```python
from build123d import *

# Parameters (mm, degrees)
SKETCH1_R           = 2.1
SKETCH1_R_2         = 6
SKETCH1_R_3         = 11
SKETCH1_R_4         = 1.6
SKETCH1_R_5         = 2
BOSS_EXTRUDE1_DEPTH = 8


with BuildPart() as part:
    # Sketch1 → Boss-Extrude1 (new body)
    with BuildSketch(Plane.XY):
        with BuildLine():
            Line((-58.658661762, -94.325772402), (11.341338238, -94.325772402))
            ThreePointArc((11.341338238, -94.325772402), (14.876872144, -92.861306308), (16.341338238, -89.325772402))
            Line((16.341338238, -89.325772402), (16.341338238, -55.206132823))
            ThreePointArc((16.341338238, -55.206132823), (18.853727353, -43.188177597), (25.970088092, -33.18314103))
            Line((25.970088092, -33.18314103), (78.712588384, 15.603630397))
            ThreePointArc((78.712588384, 15.603630397), (85.828949123, 25.608666964), (88.341338238, 37.62662219))
            Line((88.341338238, 37.62662219), (88.341338238, 93.338561628))
            ThreePointArc((88.341338238, 93.338561628), (82.483473862, 107.480697252), (68.341338238, 113.338561628))
            Line((68.341338238, 113.338561628), (46.341338238, 113.338561628))
            ThreePointArc((46.341338238, 113.338561628), (32.199202614, 107.480697252), (26.341338238, 93.338561628))
            Line((26.341338238, 93.338561628), (26.341338238, 65.996620638))
            ThreePointArc((26.341338238, 65.996620638), (23.98166612, 54.334190592), (17.273853267, 44.506394613))
            Line((17.273853267, 44.506394613), (-54.591176791, -25.493605387))
            ThreePointArc((-54.591176791, -25.493605387), (-61.298989644, -35.321401365), (-63.658661762, -46.983831411))
            Line((-63.658661762, -46.983831411), (-63.658661762, -89.325772402))
            ThreePointArc((-63.658661762, -89.325772402), (-62.194195668, -92.861306308), (-58.658661762, -94.325772402))
        make_face()
        with Locations((-56.658661762, -57.075772402)):
            Circle(SKETCH1_R, mode=Mode.SUBTRACT)
        with Locations((-30.658661762, -57.075772402)):
            Circle(SKETCH1_R, mode=Mode.SUBTRACT)
        with Locations((-30.658661762, -87.575772402)):
            Circle(SKETCH1_R, mode=Mode.SUBTRACT)
        with Locations((-56.658661762, -87.575772402)):
            Circle(SKETCH1_R, mode=Mode.SUBTRACT)
        with Locations((9.341338238, -87.575772402)):
            Circle(SKETCH1_R, mode=Mode.SUBTRACT)
        with Locations((-16.658661762, -87.575772402)):
            Circle(SKETCH1_R, mode=Mode.SUBTRACT)
        with Locations((-16.658661762, -57.075772402)):
            Circle(SKETCH1_R, mode=Mode.SUBTRACT)
        with Locations((9.341338238, -57.075772402)):
            Circle(SKETCH1_R, mode=Mode.SUBTRACT)
        with Locations((57.341338238, 99.338561628)):
            Circle(SKETCH1_R_2, mode=Mode.SUBTRACT)
        with Locations((57.341338238, 27.398561628)):
            Circle(SKETCH1_R_2, mode=Mode.SUBTRACT)
        with Locations((57.341338238, 63.368561628)):
            Circle(SKETCH1_R_3, mode=Mode.SUBTRACT)
        with Locations((41.841338238, 78.868561628)):
            Circle(SKETCH1_R_4, mode=Mode.SUBTRACT)
        with Locations((72.841338238, 78.868561628)):
            Circle(SKETCH1_R_4, mode=Mode.SUBTRACT)
        with Locations((72.841338238, 47.868561628)):
            Circle(SKETCH1_R_4, mode=Mode.SUBTRACT)
        with Locations((41.841338238, 47.868561628)):
            Circle(SKETCH1_R_4, mode=Mode.SUBTRACT)
        with Locations((84.341338238, 37.62662219)):
            Circle(SKETCH1_R_5, mode=Mode.SUBTRACT)
        with Locations((84.351781192, 88.518513838)):
            Circle(SKETCH1_R_5, mode=Mode.SUBTRACT)
        with Locations((47.341338238, 99.338561628)):
            Circle(SKETCH1_R_4, mode=Mode.SUBTRACT)
        with Locations((47.341338238, 27.398561628)):
            Circle(SKETCH1_R_4, mode=Mode.SUBTRACT)
        with Locations((67.341338238, 99.338561628)):
            Circle(SKETCH1_R_4, mode=Mode.SUBTRACT)
        with Locations((67.341338238, 27.398561628)):
            Circle(SKETCH1_R_4, mode=Mode.SUBTRACT)
        with Locations((84.346559715, 63.072568014)):
            Circle(SKETCH1_R_5, mode=Mode.SUBTRACT)
    extrude(amount=BOSS_EXTRUDE1_DEPTH)


solid = part.part
```
Source: CAD feature listing. Evaluate the final solid. Frame: model axes, mm. A direction names the side the tool comes from. Coordinates: 2 decimals unless noted, no trailing zeros. Loops run counter-clockwise (first coordinate to the right, second up) from the corner with the lowest first, then second, coordinate; pieces in that order, holes last. Notation, with made-up numbers: M -17,-11.5 L 42,-11.5 A7 cw 42,-4.5 Z; hole C 28.5,49.5 d3. An arc over 180 degrees is marked long. Put each result on its own line as item: value. Start each with the question number.
1) Cut plane B-B on x = 53.5. Return the cut outline in (y, z), then the cut area to 3 significant figures.
2) Ray query, L1, parallel to Y at x = 66, z = 3; L2, parallel to Y at x = 56, z = 5; L3, parallel to Y at x = -31.5, z = 0.5. Return the intervals inside material, ascending. Write a range as from..to.
3) Contact query for flat-ended pins moving along their axis: pin 1 Ø3 at (x, y) = (47.34, 99.34) entering from +Z; pin 2 Ø4 at (y, z) = (85, 2) entering from -X. Output: stop coordinate, or through.
4) Pull-direction query (X, two-part tool) for faces 1 (the face through (52.919, 103.394, 3.944)), 2 (the face through (11, 11, 0)), 3 (the face through (-63.659, -68, 4)); classes: pulls with the +X half, pulls with the -X half, needs draft (parallel to the pull), parting line crosses it, or undercut.
5) Cut plane D-D on z = 6.5. Give the number of separate pieces and of enclosed holes in the cut face, then the cut area to 3 significant figures.
6) Reachability of faces 4 (the face through (26.341, 80, 4)), 5 (the face through (83.91, 61.12, 3.94)) from +Z, -Z, +X, -X, +Y, -Y: full face, straight path, thin tool, end or side. Return the list, or none.
7) Cut plane A-A on y = 70.5. Return the cut outline in (x, z).
8) Cut plane C-C on y = -71. Return the cut outline in (x, z).
The answers:
1. outline: M -7.72,0 L 22.79,0 L 22.79,8 L -7.72,8 Z; M 32.01,0 L 53.06,0 L 53.06,8 L 32.01,8 Z; M 73.68,0 L 94.73,0 L 94.73,8 L 73.68,8 Z; M 103.95,0 L 113.34,0 L 113.34,8 L 103.95,8 Z
1. area: 656 mm²
2. L1: y = 3.84..26.53, 28.27..56.58, 70.15..98.47, 100.21..113.34
2. L2: y = -5.41..21.55, 33.25..52.45, 74.29..93.49, 105.19..113.34
2. L3: y = -94.33..-89.5, -85.65..-59, -55.15..-3
3. pin 1: passes through
3. pin 2: stops at x = 26.34
4. face 1: undercut
4. face 2: needs draft
4. face 3: pulls with the -X half
5. separate pieces: 1
5. enclosed holes: 22
5. area: 15,100 mm²
6. face 4: +Z, -Z, -X, +Y
6. face 5: +Z, -Z
7. outline: M 26.34,0 L 48.97,0 L 48.97,8 L 26.34,8 Z; M 65.72,0 L 88.34,0 L 88.34,8 L 65.72,8 Z
8. outline: M -63.66,0 L 16.34,0 L 16.34,8 L -63.66,8 Z
